Verification items for this drawing (mm, ordinates from the low corner). A direction names the side the tool comes from. Coordinates: 2 decimals unless noted, no trailing zeros. Order: outer loops, then holes, each group sorted by start corner. A loop starts at its lowest first (then second) coordinate and runs counter-clockwise, first axis right, second up. Notation, with made-up numbers: (42.5, -14.75) - (76.5, -14.75) arc R16 ccw to (76.5, 0.25) - close; hole circle Ø2 at (83.25, -26). An arc over 180 degrees is marked (long way). Use CSV: the item, a comma, the result in double quotes. Start each with the question number.
1) Sectioned sample at D-D, the plane x = 12.75. Record the cut outline in (y, z).
2) Sectioned sample at C-C, the plane z = 3.5. Record the cut outline in (x, y), and give its area (3 significant figures).
3) Tool access check on the marked faces 1, 2 and 3. Record the directions out of +Z, -Z, +X, -X, +Y, -Y that give a thin tool (end or side, any length) a straight path to the whole face; none if there is none.
4) Thickness scan on probe 1 along Z at (x, y) = (11.25, 0.5); probe 2 along X at (y, z) = (3.6, 11.25); probe 3 along X at (y, z) = (0.6, 8). Record the ranges inside material, lowest first. Write a range as [from, to].
5) Sectioned sample at B-B, the plane y = 2.75. Record the cut outline in (x, z), and give its area (4 significant figures).
6) Sectioned sample at A-A, the plane x = 1.75. Record the cut outline in (y, z).
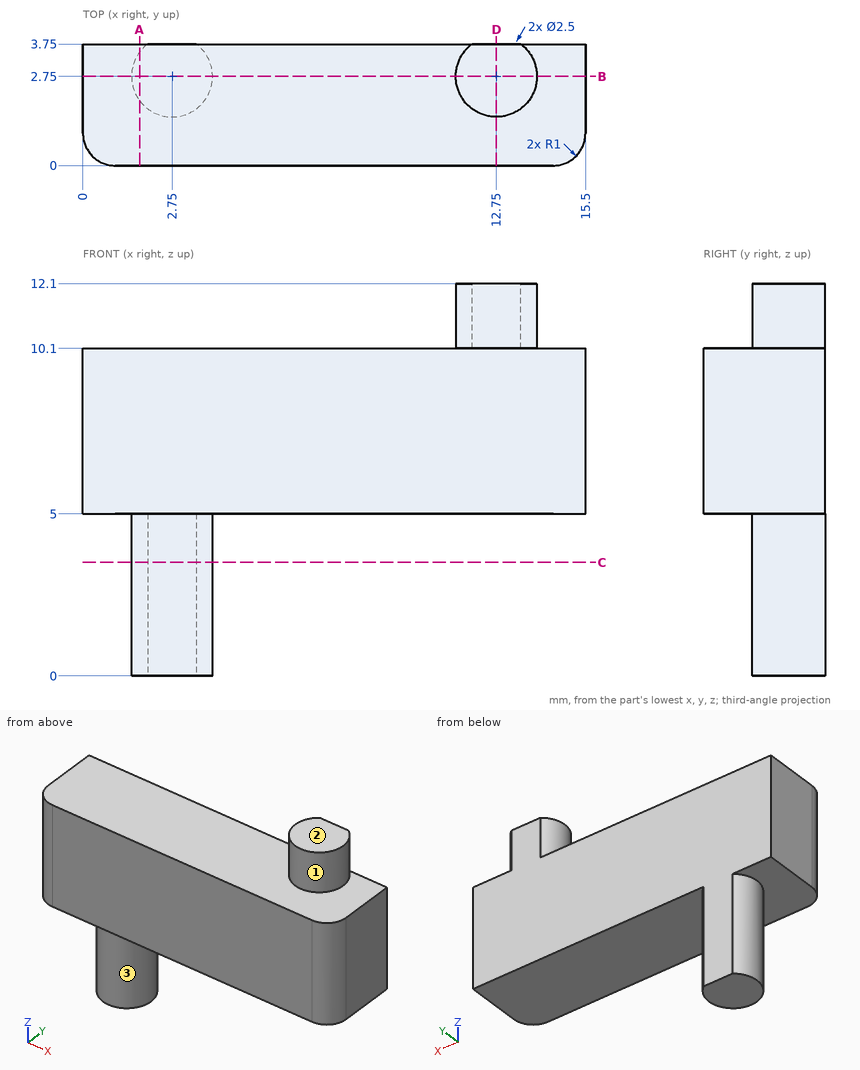
Evaluation:
1,outline,"(0, 5) - (3.75, 5) - (3.75, 12.1) - (1.5, 12.1) - (1.5, 10.1) - (0, 10.1) - close"
2,outline,"(2, 3.75) arc R1.25 ccw (long way) to (3.5, 3.75) - close"
2,area,"4.65 mm²"
3,face 1,"+Z"
3,face 2,"+Z, +X, -X, +Y, -Y"
3,face 3,"-Z"
4,probe 1,"[5, 10.1]"
4,probe 2,"[11.83, 13.67]"
4,probe 3,"[0.08, 15.42]"
5,outline,"(0, 5) - (1.5, 5) - (1.5, 0) - (4, 0) - (4, 5) - (15.5, 5) - (15.5, 10.1) - (14, 10.1) - (14, 12.1) - (11.5, 12.1) - (11.5, 10.1) - (0, 10.1) - close"
5,area,"96.55 mm²"
6,outline,"(0, 5) - (2, 5) - (2, 0) - (3.5, 0) - (3.5, 5) - (3.75, 5) - (3.75, 10.1) - (0, 10.1) - close"
